```python
from build123d import *

# Parameters (mm, degrees)
SKETCH1_W               = 50.8
SKETCH1_H               = 76.2
SKETCH1_W_2             = 44.45
SKETCH1_H_2             = 69.85
BOSS_EXTRUDE1_DEPTH     = 95
CUT_EXTRUDE2_DEPTH      = 106.459802769
CUT_EXTRUDE2_DEPTH_BACK = 106.459802769
SKETCH3_R               = 5
SKETCH3_W               = 95
SKETCH3_H               = 24.975
SKETCH3_W_2             = 60
SKETCH3_H_2             = 20
FILLET2_R               = 6.35


with BuildPart() as part:
    # Sketch1 → Boss-Extrude1 (new body)
    with BuildSketch(Plane.XY):
        Rectangle(SKETCH1_W, SKETCH1_H)
        Rectangle(SKETCH1_W_2, SKETCH1_H_2, mode=Mode.SUBTRACT)
    extrude(amount=BOSS_EXTRUDE1_DEPTH)

    # Sketch3 → Cut-Extrude2 (cut, two sides: drawn at the far end of the back side and taken through both)
    with BuildSketch(Plane(origin=(0, 0, 0), x_dir=(0, 0, -1), z_dir=(1, 0, 0)).offset(-CUT_EXTRUDE2_DEPTH_BACK)):
        with Locations((-86.875, -5)):
            Circle(SKETCH3_R)
        with Locations(Location((-8.125, -5, 0), (0, 0, 270))):
            Circle(SKETCH3_R)
        with Locations((-47.5, -25.6125)):
            Rectangle(SKETCH3_W, SKETCH3_H)
        with Locations((-47.5, 15.925)):
            Rectangle(SKETCH3_W_2, SKETCH3_H_2)
    extrude(amount=CUT_EXTRUDE2_DEPTH + CUT_EXTRUDE2_DEPTH_BACK, mode=Mode.SUBTRACT)

    # Fillet2
    fillet2_edges = [part.edges().sort_by_distance(p)[0] for p in [
        (-23.8125, 25.925, 17.5),
        (-23.8125, 5.925, 17.5),
        (-23.8125, 5.925, 77.5),
        (-23.8125, 25.925, 77.5),
        (23.8125, 25.925, 17.5),
        (23.8125, 5.925, 17.5),
        (23.8125, 5.925, 77.5),
        (23.8125, 25.925, 77.5),
    ]]
    fillet(fillet2_edges, radius=FILLET2_R)


solid = part.part
```
Model file for the job. Use its own axes, mm. A direction names the side the tool comes from. Give positions to 0.01 mm unless a question says otherwise; leave off trailing zeros. Order: outer loops, then holes, each group sorted by start corner. A loop starts at its lowest first (then second) coordinate and runs counter-clockwise, first axis right, second up.
1) Mould opens along Z. For faces 4 (the cylindrical face through (-23.79, 7.835, 75.689)), 5 (the flat face through (-24, -13.125, 48)), 6 (the flat face through (-3.9, 35.4, 0)) say: +Z half, -Z half, draft (parallel to the pull), parting line (faces both ways), or undercut.
2) Wall check: probe 1 along Z at (x, y) = (-23.95, -5) (3 decimals); probe 2 along X at (y, z) = (-4, 66) (3 decimals); probe 3 along Y at (x, z) = (17, 72) (3 decimals). Give the ranges that are in metal, low to high.
3) Saw through at D-D, the plane x = 4.5. Write the cut outline in (y, z) (3 decimals).
4) Saw through at A-A, the plane y = 31.5. Write the cut outline in (x, z) (3 decimals).
5) Saw through at B-B, the plane z = 50.5. Write the cut outline in (x, y) (3 decimals), then the cut area to 3 significant figures.
6) Saw through at C-C, the plane y = -5. Write the cut outline in (x, z) (3 decimals).
7) Pin check, flat tip, straight feed: pin 1 (6 mm diameter, centred on x = -12.5, z = 11.5, fed in from -Y) (3 decimals). Stop position of the tip, or through.
8) 3-axis set-ups, long thin cutter, end or side, ignore diameter. For faces 1 (the flat face through (24, 16, 17.5)), 2 (the flat face through (0, 34.925, 47)), 3 (the flat face through (-3.9, 35.4, 95)): which of +Z, -Z, +X, -X, +Y, -Y reach the whole face in a straight line?
Computed:
1. face 4: undercut
1. face 5: draft
1. face 6: -Z half
2. probe 1: z = 0 to 3.125, 13.125 to 81.875, 91.875 to 95
2. probe 2: x = -25.4 to -22.225, 22.225 to 25.4
2. probe 3: y = 34.925 to 38.1
3. outline: (34.925, 0) - (38.1, 0) - (38.1, 95) - (34.925, 95) - close
4. outline: (-25.4, 0) - (-22.225, 0) - (-22.225, 95) - (-25.4, 95) - close; (22.225, 0) - (25.4, 0) - (25.4, 95) - (22.225, 95) - close
5. outline: (-25.4, -13.125) - (-22.225, -13.125) - (-22.225, 5.925) - (-25.4, 5.925) - close; (-25.4, 25.925) - (-22.225, 25.925) - (-22.225, 34.925) - (22.225, 34.925) - (22.225, 25.925) - (25.4, 25.925) - (25.4, 38.1) - (-25.4, 38.1) - close; (22.225, -13.125) - (25.4, -13.125) - (25.4, 5.925) - (22.225, 5.925) - close
5. area: 339 mm2
6. outline: (-25.4, 0) - (-22.225, 0) - (-22.225, 3.125) - (-25.4, 3.125) - close; (-25.4, 13.125) - (-22.225, 13.125) - (-22.225, 81.875) - (-25.4, 81.875) - close; (-25.4, 91.875) - (-22.225, 91.875) - (-22.225, 95) - (-25.4, 95) - close; (22.225, 0) - (25.4, 0) - (25.4, 3.125) - (22.225, 3.125) - close; (22.225, 13.125) - (25.4, 13.125) - (25.4, 81.875) - (22.225, 81.875) - close; (22.225, 91.875) - (25.4, 91.875) - (25.4, 95) - (22.225, 95) - close
7. pin 1: stops at y = 34.925
8. face 1: +X, -X
8. face 2: +Z, -Z, -Y
8. face 3: +Z, +X, -X, +Y, -Y
